from build123d import *

# Parameters (mm, degrees)
F0_R            = 63.5
F1_DEPTH        = 6.35
F3_DEPTH        = 12.7
F3_COPIES_COUNT = 25


# Not quite as in the source:
# - a pattern or mirror of a feature is missing from the dataset's text; its kind, count and spacing are read off the source's solid


with BuildPart() as f1:
    # F0 (on Top) → F1 (new body, symmetric)
    with BuildSketch(Plane.XY):
        Circle(F0_R)
    extrude(amount=F1_DEPTH, both=True)

    # F2 (on face) → F3 (join, through all)
    with BuildSketch(Plane.XY.offset(6.35)):
        with BuildLine():
            Line((0, 78.9130567023), (-7.9355522703, 63.002198455))
            ThreePointArc((-7.9355522703, 63.002198455), (0, 63.5), (7.9355522703, 63.002198455))
            Line((7.9355522703, 63.002198455), (0, 78.9130567023))
        make_face()
    f3 = extrude(amount=-F3_DEPTH)

    # F3_copies: F3 ×25 about axis
    f3_copies_axis = Axis((0, 0, 0), (0, 0, 1))
    for i in range(1, F3_COPIES_COUNT):
        add(f3.rotate(f3_copies_axis, i * 360 / F3_COPIES_COUNT))


solid = f1.part
For this review, take the finished solid that the model builds, in its own axes (mm). A direction names the side the tool comes from. Coordinates: 2 decimals unless noted, no trailing zeros. Write each loop counter-clockwise with the first axis right and the second up, starting at its lowest first coordinate (ties: lowest second). Pieces come first, ordered by that corner, then holes. Notation, with made-up numbers: (-38, 29.25) -> (-34, 29.25) arc R33 cw to (-34, 68.25) -> close; hole circle Ø4 at (56, 20.5). An arc over 180 degrees is marked (long way). Write each question's results on one line, items separated by ' | '. Start each with the question number.
1) Wall thickness on L1, parallel to Y at x = 65, z = -5; L2, parallel to X at y = -58, z = 0.75; L3, parallel to X at y = 64, z = -5.25: over which ranges is each line inside the solid? List them lowest first. Write a range as [from, to].
2) Consider section B-B (y = 35.5). Write out the cut boundary in (x, z).
3) The part is to be moulded in two halves that separate along Y. For faces 1 (the face through (-1, 1, -6.35)), 2 (the face through (-66.14, 25.72, 0.09)), 3 (the face through (-29.82, -64.39, 0.09)), say which applies: +Y half, -Y half, draft (parallel to the pull), parting line (faces both ways), or undercut.
4) Consider section A-A (y = 54). Write out the cut boundary in (x, z).
5) Insertion check: pin 1 (6 mm diameter, centred on y = 13, z = 2, fed in from -X); pin 2 (2 mm diameter, centred on y = -41.5, z = -2.5, fed in from +X); pin 3 (3 mm diameter, centred on y = 35, z = 2, fed in from -X). Each pin has a flat end and moves straight along its axis. Give the tip position at first contact, or say it passes through.
6) For faces 4 (the face through (4.888, -70.792, 0.089)), 5 (the face through (57.253, -42.287, 0.089)), 6 (the face through (-13.72, 69.62, 0.09)), 7 (the face through (52.02, -48.26, 0.09)), list the 3-axis set-ups (+Z, -Z, +X, -X, +Y, -Y) from which the entire face can be reached by the end or side of a thin tool; tool diameter is ignored.
Geometry says:
1) L1: [-33.75, -25.49], [-18.31, -5.25], [-3.02, 10.77], [14.51, 25.89], [39.58, 42.12] | L2: [-45.41, -35.16], [-30.37, 30.37], [35.16, 45.41] | L3: [-37.81, -30.57], [-22.29, -8.85], [-7.44, 7.44], [8.85, 22.29], [30.57, 37.81]
2) outline: (-62.54, -6.35) -> (62.54, -6.35) -> (62.54, 6.35) -> (-62.54, 6.35) -> close
3) face 1: draft | face 2: undercut | face 3: -Y half
4) outline: (-52.96, -6.35) -> (-44.49, -6.35) -> (-44.49, 6.35) -> (-52.96, 6.35) -> close; (-37.41, -6.35) -> (37.41, -6.35) -> (37.41, 6.35) -> (-37.41, 6.35) -> close; (44.49, -6.35) -> (52.96, -6.35) -> (52.96, 6.35) -> (44.49, 6.35) -> close
5) pin 1: x = -66.82 | pin 2: x = 57.35 | pin 3: x = -63.14
6) face 4: +Z, -Z, -Y | face 5: +Z, -Z, +X | face 6: +Z, -Z, +Y | face 7: +Z, -Z
